For this review, take the finished solid that the model builds, in its own axes (mm). Face numbers are marked on the shaded views. A direction names the side the tool comes from. Coordinates: 2 decimals unless noted, no trailing zeros. Loops run counter-clockwise (first coordinate to the right, second up) from the corner with the lowest first, then second, coordinate; pieces in that order, holes last. Notation, with made-up numbers: (3, 70) - (22, 70) arc R22 cw to (22, 78) - close; hole circle Ø6 at (-25.75, 26). An arc over 180 degrees is marked (long way). Answer as a JSON object with one key per item and string values. Group by question number.
Item 1: We need section C-C (x = 40.5). Give the boundary of the cut face in (y, z).
Item 2: We need section D-D (y = 10.5). Give the boundary of the cut face in (x, z), then the cut area to 3 significant figures.
Item 3: We need section B-B (z = 16.5). Give the boundary of the cut face in (x, y), then the cut area to 3 significant figures.
Item 4: Tool access review of the marked faces 1, 2 and 3: name each direction out of +Z, -Z, +X, -X, +Y, -Y from which nothing blocks a thin tool from reaching the whole face with its end or side.
Item 5: To check wall thickness, follow line 1 (Y direction, x = 39.5, z = 14); line 2 (Z direction, x = 45, y = -9.5); line 3 (Z direction, x = 27, y = -10.5). State the ranges of each line that lie inside material, in increasing order.
Item 6: We need section A-A (y = -12). Give the boundary of the cut face in (x, z), then the cut area to 3 significant figures.
Item 7: Clearance check with flat-ended pins moving along their axes: pin 1 (9.5 mm diameter, centred on x = 6, z = 10, fed in from -Y); pin 2 (6 mm diameter, centred on x = 28, z = 6.5, fed in from -Y); pin 3 (9.5 mm diameter, centred on x = 5, y = -6, fed in from +Z). State where each tip first meets the part, or that it passes through.
from build123d import *

# Parameters (mm, degrees)
F1_DEPTH = 50.8
F3_DEPTH = 25.4
F4_W     = 12.7
F4_H     = 19.05
F5_DEPTH = 19.05
F7_DEPTH = 25.4


with BuildPart() as f1:
    # F0 (on Right) → F1 (new body)
    with BuildSketch(Plane.YZ):
        Polygon((0, 19.05), (0, 0), (-19.05, 0), (-19.05, -12.7), (12.7, -12.7), (12.7, 19.05), align=None)
    extrude(amount=F1_DEPTH)

    # F2 (on face) → F3 (cut)
    with BuildSketch(Plane.XZ):
        Polygon((50.8, 0), (50.8, 19.05), (44.45, 19.05), align=None)
    extrude(amount=-F3_DEPTH, mode=Mode.SUBTRACT)

    # F4 (on face) → F5 (join)
    with BuildSketch(Plane.XZ):
        with Locations((25.4, 9.525)):
            Rectangle(F4_W, F4_H)
    extrude(amount=F5_DEPTH)

    # F6 (on face) → F7 (cut)
    with BuildSketch(Plane.YZ.offset(31.75)):
        Polygon((-19.05, 19.05), (-19.05, 0), (0, 19.05), align=None)
    extrude(amount=-F7_DEPTH, mode=Mode.SUBTRACT)


solid = f1.part
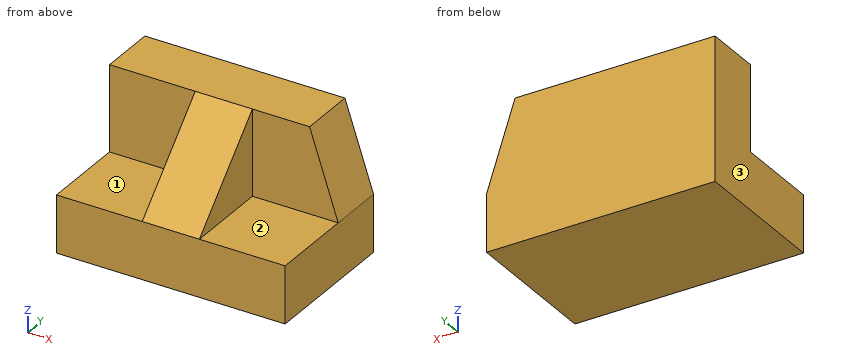
Check sheet entries:
{
 "1": {"outline": "(-19.05, -12.7) - (12.7, -12.7) - (12.7, 19.05) - (0, 19.05) - (0, 0) - (-19.05, 0) - close"},
 "2": {"outline": "(0, -12.7) - (50.8, -12.7) - (50.8, 0) - (44.45, 19.05) - (0, 19.05) - close", "area": "1,550 mm2"},
 "3": {"outline": "(0, 0) - (19.05, 0) - (19.05, -2.55) - (31.75, -2.55) - (31.75, 0) - (45.3, 0) - (45.3, 12.7) - (0, 12.7) - close", "area": "608 mm2"},
 "4": {"face 1": "+Z, -X, -Y", "face 2": "+Z, +X, -Y", "face 3": "+Z, -Z, -X, +Y, -Y"},
 "5": {"line 1": "y = 0 to 12.7", "line 2": "z = -12.7 to 0", "line 3": "z = -12.7 to 8.55"},
 "6": {"outline": "(0, -12.7) - (50.8, -12.7) - (50.8, 0) - (31.75, 0) - (31.75, 7.05) - (19.05, 7.05) - (19.05, 0) - (0, 0) - close", "area": "735 mm2"},
 "7": {"pin 1": "stops at y = 0", "pin 2": "stops at y = -15.55", "pin 3": "stops at z = 0"}
}
